```python
from build123d import *

# Parameters (mm, degrees)
BOSS_EXTRUDE1_DEPTH        = 5
BOSS_EXTRUDE2_DEPTH        = 5
SKETCH10_W                 = 7
SKETCH10_H                 = 7
CUT_EXTRUDE2_DEPTH         = 2.6
SKETCH11_R                 = 2.1
CUT_EXTRUDE3_DEPTH         = 37.99114612
F_3_2_3_2_DIAMETER_HOLE1_D = 3.2


with BuildPart() as part:
    # Sketch1 → Boss-Extrude1 (new body)
    with BuildSketch(Plane(origin=(0, 0, 0), x_dir=(1, 0, 0), z_dir=(0, 1, 0))):
        with BuildLine():
            Line((-196.961550602, 34.729635533), (-187.113473072, 32.993153757))
            ThreePointArc((-187.113473072, 32.993153757), (-190, 0), (-187.113473072, -32.993153757))
            Line((-187.113473072, -32.993153757), (-196.961550602, -34.729635533))
            ThreePointArc((-196.961550602, -34.729635533), (-200, 0), (-196.961550602, 34.729635533))
        make_face()
    extrude(amount=BOSS_EXTRUDE1_DEPTH)

    # Sketch9 → Boss-Extrude2 (add)
    with BuildSketch(Plane(origin=(0, 5, 0), x_dir=(1, 0, 0), z_dir=(0, 1, 0))):
        with BuildLine():
            Line((-199.749843554, 10), (-189.73665961, 10))
            ThreePointArc((-189.73665961, 10), (-190, 0), (-189.73665961, -10))
            Line((-189.73665961, -10), (-199.749843554, -10))
            ThreePointArc((-199.749843554, -10), (-200, 0), (-199.749843554, 10))
        make_face()
    extrude(amount=BOSS_EXTRUDE2_DEPTH)

    # Sketch10 → Cut-Extrude2 (cut)
    with BuildSketch(Plane.ZY.offset(195)):
        with Locations((0, 10)):
            Rectangle(SKETCH10_W, SKETCH10_H)
    extrude(amount=-CUT_EXTRUDE2_DEPTH, mode=Mode.SUBTRACT)

    # Sketch11 → Cut-Extrude3 (cut, through all)
    with BuildSketch(Plane.ZY.offset(195)):
        with Locations((0, 10)):
            Circle(SKETCH11_R)
    extrude(amount=-CUT_EXTRUDE3_DEPTH, mode=Mode.SUBTRACT)

    # Ø3.2 (3.2) Diameter Hole1 (through all)
    with Locations(Plane(origin=(0, 5, 0), x_dir=(1, 0, 0), z_dir=(0, 1, 0))):
        with Locations((-194.257966128, 16.995369836), (-193.331747968, 25.452607483), (-194.257966128, -16.995369836), (-193.331747968, -25.452607483)):
            Hole(F_3_2_3_2_DIAMETER_HOLE1_D / 2)


solid = part.part
```
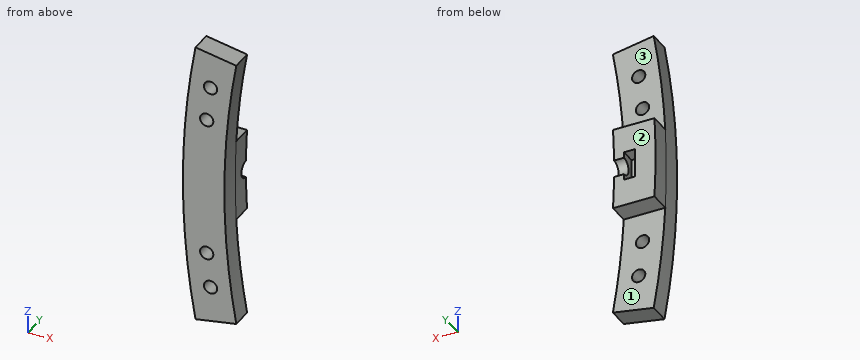
Geometry check sheet. Reference: the model listing, model coordinates, mm. Face numbers are marked on the shaded views. A direction names the side the tool comes from. Give positions to 0.01 mm unless a question says otherwise; leave off trailing zeros. Order: outer loops, then holes, each group sorted by start corner. A loop starts at its lowest first (then second) coordinate and runs counter-clockwise, first axis right, second up. Notation, with made-up numbers: (-35.5, -1) -> (7.5, -1) arc R4 cw to (7.5, 5) -> close; hole circle Ø7 at (-14, 37.25). An arc over 180 degrees is marked (long way). Write each question's results on one line, items separated by ' | '. Start each with the question number.
(1) Sectioned sample at C-C (y = 3.5). Enter the section's corners in (x, z), plus the area to 3 significant figures.
(2) Gauge pin test, flat ends, axial feed: P1, Ø3, axis at y = 9, z = -0.5, coming from the -X side; P2, Ø2, axis at y = 5.5, z = -26, coming from the -X side; P3, Ø2.5, axis at x = -192.5, y = 8.5, coming from the +Z side; P4, Ø2, axis at x = -190, z = 22.5, coming from the -Y side. Record the tip position at first contact, or that the pin passes through.
(3) Sectioned sample at A-A (x = -188.75). Enter the section's corners in (y, z).
(4) Sectioned sample at B-B (z = 0). Enter the section's corners in (x, y).
(5) Scan lines: line 1 (Z direction, x = -192.5, y = 2.5); line 2 (Z direction, x = -192, y = 1.25); line 3 (Z direction, x = -194.25, y = 7). Record each from-to range of solid material in increasing order.
(6) Access from +Z, -Z, +X, -X, +Y, -Y to the whole of each face (thin tool, end or side, straight path). Record for the marked faces 1, 2 and 3.
(7) Sectioned sample at D-D (z = 11.5). Enter the section's corners in (x, y).
Answer below:
1) outline: (-196.96, -34.73) -> (-187.11, -32.99) arc R190 cw to (-187.11, 32.99) -> (-196.96, 34.73) arc R200 ccw to start; hole circle Ø3.2 at (-194.26, -17); hole circle Ø3.2 at (-194.26, 17); hole circle Ø3.2 at (-193.33, -25.45); hole circle Ø3.2 at (-193.33, 25.45) | area: 649 mm2
2) P1: x = -200 | P2: x = -198.41 | P3: z = 10 | P4: y = 0
3) outline: (0, -33.28) -> (5, -33.28) -> (5, -21.76) -> (0, -21.76) -> close; (0, 21.76) -> (5, 21.76) -> (5, 33.28) -> (0, 33.28) -> close
4) outline: (-200, 0) -> (-190, 0) -> (-190, 7.9) -> (-192.4, 7.9) -> (-192.4, 6.5) -> (-195, 6.5) -> (-195, 10) -> (-200, 10) -> close
5) line 1: -33.94 to -26.82, -24.09 to 24.09, 26.82 to 33.94 | line 2: -33.85 to -26.34, -24.57 to 24.57, 26.34 to 33.85 | line 3: -10 to -3.5, 3.5 to 10
6) face 1: -Z, +X, -X, +Y | face 2: +Z, -Z, +X, -X, +Y | face 3: +Z, +X, -X, +Y
7) outline: (-199.67, 0) -> (-189.65, 0) -> (-189.65, 5) -> (-199.67, 5) -> close
